Source: CAD feature listing. Evaluate the final solid. Frame: model axes, mm. Coordinates: 2 decimals unless noted, no trailing zeros. Order: outer loops, then holes, each group sorted by start corner. A loop starts at its lowest first (then second) coordinate and runs counter-clockwise, first axis right, second up. Notation, with made-up numbers: (-2, 61.25) -> (32, 61.25) arc R24 cw to (32, 73.25) -> close; hole circle Ø3 at (-23.75, 1). An arc over 180 degrees is marked (long way). Write each question's results on one line, items separated by ' | '. Start each with the question number.
from build123d import *

# Parameters (mm, degrees)
SKETCH1_W           = 56
SKETCH1_H           = 88.9
SKETCH1_R           = 2.1
BOSS_EXTRUDE1_DEPTH = 4
FILLET1_R           = 4


with BuildPart() as part:
    # Sketch1 → Boss-Extrude1 (new body)
    with BuildSketch(Plane(origin=(0, 0, 0), x_dir=(1, 0, 0), z_dir=(0, 1, 0))):
        with Locations((0, -36.45)):
            Rectangle(SKETCH1_W, SKETCH1_H)
        with Locations(Location((-16, 0, 0), (0, 0, 270))):
            Circle(SKETCH1_R, mode=Mode.SUBTRACT)
        with Locations(Location((16, 0, 0), (0, 0, 270))):
            Circle(SKETCH1_R, mode=Mode.SUBTRACT)
        with Locations(Location((-8, 0, 0), (0, 0, 270))):
            Circle(SKETCH1_R, mode=Mode.SUBTRACT)
        with Locations(Location((0, 0, 0), (0, 0, 270))):
            Circle(SKETCH1_R, mode=Mode.SUBTRACT)
        with Locations(Location((8, 0, 0), (0, 0, 270))):
            Circle(SKETCH1_R, mode=Mode.SUBTRACT)
        with Locations(Location((-16, -16, 0), (0, 0, 270))):
            Circle(SKETCH1_R, mode=Mode.SUBTRACT)
        with Locations(Location((-8, -16, 0), (0, 0, 270))):
            Circle(SKETCH1_R, mode=Mode.SUBTRACT)
        with Locations(Location((0, -16, 0), (0, 0, 270))):
            Circle(SKETCH1_R, mode=Mode.SUBTRACT)
        with Locations(Location((8, -16, 0), (0, 0, 270))):
            Circle(SKETCH1_R, mode=Mode.SUBTRACT)
        with Locations(Location((16, -16, 0), (0, 0, 270))):
            Circle(SKETCH1_R, mode=Mode.SUBTRACT)
        with Locations(Location((-16, -32, 0), (0, 0, 270))):
            Circle(SKETCH1_R, mode=Mode.SUBTRACT)
        with Locations(Location((-8, -32, 0), (0, 0, 270))):
            Circle(SKETCH1_R, mode=Mode.SUBTRACT)
        with Locations(Location((0, -32, 0), (0, 0, 270))):
            Circle(SKETCH1_R, mode=Mode.SUBTRACT)
        with Locations(Location((8, -32, 0), (0, 0, 270))):
            Circle(SKETCH1_R, mode=Mode.SUBTRACT)
        with Locations(Location((16, -32, 0), (0, 0, 270))):
            Circle(SKETCH1_R, mode=Mode.SUBTRACT)
        with Locations(Location((-16, -48, 0), (0, 0, 270))):
            Circle(SKETCH1_R, mode=Mode.SUBTRACT)
        with Locations(Location((-8, -48, 0), (0, 0, 270))):
            Circle(SKETCH1_R, mode=Mode.SUBTRACT)
        with Locations(Location((0, -48, 0), (0, 0, 270))):
            Circle(SKETCH1_R, mode=Mode.SUBTRACT)
        with Locations(Location((8, -48, 0), (0, 0, 270))):
            Circle(SKETCH1_R, mode=Mode.SUBTRACT)
        with Locations(Location((16, -48, 0), (0, 0, 270))):
            Circle(SKETCH1_R, mode=Mode.SUBTRACT)
        with Locations(Location((-16, -64, 0), (0, 0, 270))):
            Circle(SKETCH1_R, mode=Mode.SUBTRACT)
        with Locations(Location((-8, -64, 0), (0, 0, 270))):
            Circle(SKETCH1_R, mode=Mode.SUBTRACT)
        with Locations(Location((0, -64, 0), (0, 0, 270))):
            Circle(SKETCH1_R, mode=Mode.SUBTRACT)
        with Locations(Location((8, -64, 0), (0, 0, 270))):
            Circle(SKETCH1_R, mode=Mode.SUBTRACT)
        with Locations(Location((16, -64, 0), (0, 0, 270))):
            Circle(SKETCH1_R, mode=Mode.SUBTRACT)
    extrude(amount=BOSS_EXTRUDE1_DEPTH)

    # Fillet1
    fillet1_edges = [part.edges().sort_by_distance(p)[0] for p in [
        (-28, 2, -8),
        (28, 2, -8),
        (28, 2, 80.9),
        (-28, 2, 80.9),
    ]]
    fillet(fillet1_edges, radius=FILLET1_R)


solid = part.part
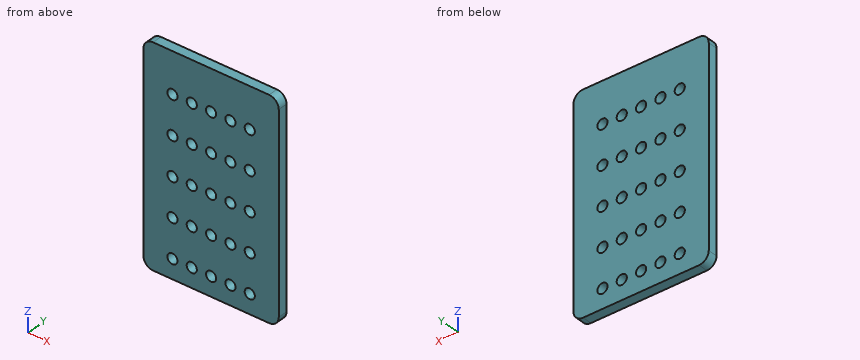
(1) Section A-A on x = -16. Return the cut outline in (y, z), then the cut area to 3 significant figures.
(2) Section B-B on z = 64. Return the cut outline in (x, y).
(3) Line query: L1, parallel to X at y = 2.9, z = 16; L2, parallel to X at y = 1.4, z = 17.5; L3, parallel to Z at x = -15, y = 1.7. Output: solid intervals per line, ascending.
(4) First-contact query: P1, Ø2.5, axis at x = 0, z = 48, coming from the +Y side; P2, Ø5, axis at x = 19, z = 41.5, coming from the -Y side. Flat tips, straight axial feed; report the tip coordinate or a pass-through.
(5) Section C-C on y = 3. Count the separate pieces of the cut face and the enclosed holes in it, then the cut area to 3 significant figures.
Results list:
1) outline: (0, -8) -> (4, -8) -> (4, -2.1) -> (0, -2.1) -> close; (0, 2.1) -> (4, 2.1) -> (4, 13.9) -> (0, 13.9) -> close; (0, 18.1) -> (4, 18.1) -> (4, 29.9) -> (0, 29.9) -> close; (0, 34.1) -> (4, 34.1) -> (4, 45.9) -> (0, 45.9) -> close; (0, 50.1) -> (4, 50.1) -> (4, 61.9) -> (0, 61.9) -> close; (0, 66.1) -> (4, 66.1) -> (4, 80.9) -> (0, 80.9) -> close | area: 272 mm²
2) outline: (-28, 0) -> (-18.1, 0) -> (-18.1, 4) -> (-28, 4) -> close; (-13.9, 0) -> (-10.1, 0) -> (-10.1, 4) -> (-13.9, 4) -> close; (-5.9, 0) -> (-2.1, 0) -> (-2.1, 4) -> (-5.9, 4) -> close; (2.1, 0) -> (5.9, 0) -> (5.9, 4) -> (2.1, 4) -> close; (10.1, 0) -> (13.9, 0) -> (13.9, 4) -> (10.1, 4) -> close; (18.1, 0) -> (28, 0) -> (28, 4) -> (18.1, 4) -> close
3) L1: x = -28 to -18.1, -13.9 to -10.1, -5.9 to -2.1, 2.1 to 5.9, 10.1 to 13.9, 18.1 to 28 | L2: x = -28 to -17.47, -14.53 to -9.47, -6.53 to -1.47, 1.47 to 6.53, 9.47 to 14.53, 17.47 to 28 | L3: z = -8 to -1.85, 1.85 to 14.15, 17.85 to 30.15, 33.85 to 46.15, 49.85 to 62.15, 65.85 to 80.9
4) P1: passes through | P2: stops at y = 0
5) separate pieces: 1 | enclosed holes: 25 | area: 4,620 mm²
